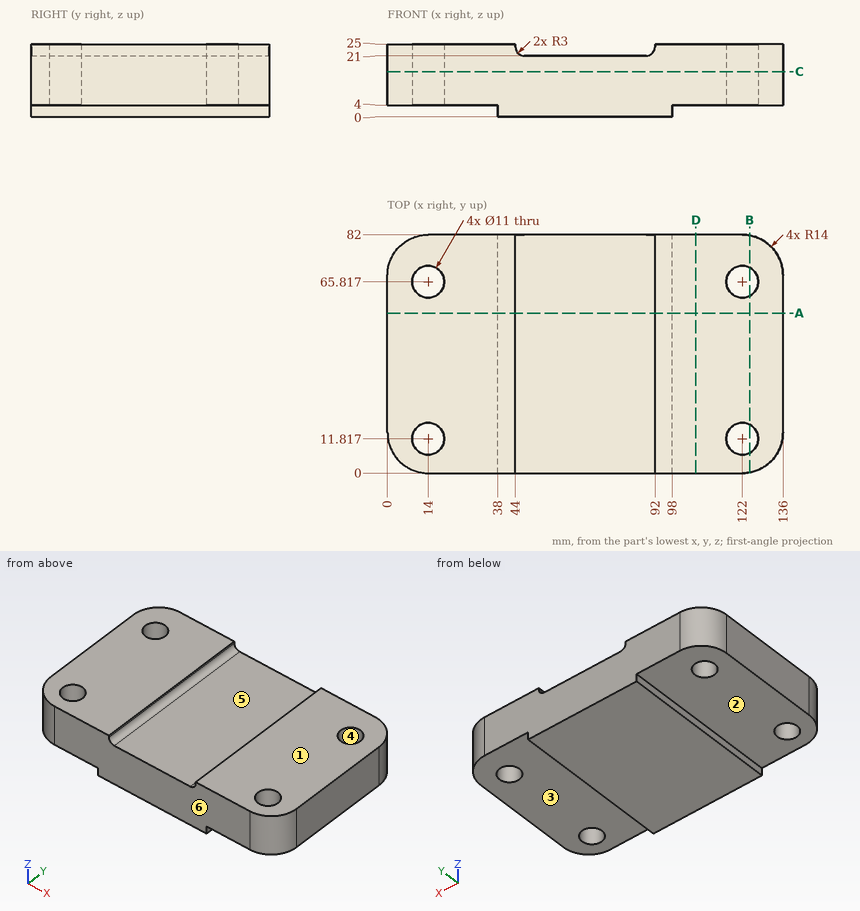
Could you check a few things on this drawing? It's one solid part, dimensions in mm from its lowest x, y, z. A direction names the side the tool comes from. Coordinates: 2 decimals unless noted, no trailing zeros. Order: outer loops, then holes, each group sorted by start corner. A loop starts at its lowest first (then second) coordinate and runs counter-clockwise, first axis right, second up. Notation, with made-up numbers: M -34,88 L -24,88 A33 ccw -24,121 Z; hole C 63.25,-14.75 d3. An arc over 180 degrees is marked long. Use a Markdown table: item, result. Add a question column.
Q1. I'm going to push flat-ended pins straight in: pin 1 (2 mm diameter, centred on y = 22, z = 2, fed in from -X); pin 2 (2 mm diameter, centred on x = 17.5, y = 53, fed in from -Z); pin 3 (1.2 mm diameter, centred on y = 36, z = 1.5, fed in from +X). Where does each tip first touch, or does it pass through?
Q2. I want a section at B-B on x = 124.5. List the corners of the cut face in (y, z) for me (1 decimal).
Q3. I want a section at C-C on z = 15.5. List the corners of the cut face in (x, y) for me.
Q4. We'd pull the mould along Y, two halves only. Please class the marked faces 4, 5 and 6: pulls with the +Y half, pulls with the -Y half, needs draft (parallel to the pull), parting line crosses it, or undercut.
Q5. I want a section at D-D on x = 106. List the corners of the cut face in (y, z) for me.
Q6. I want a section at A-A on y = 55. List the corners of the cut face in (x, z) for me, then the cut area to 3 significant figures.
Q7. Which directions (+Z, -Z, +X, -X, +Y, -Y) give clear straight access to the entire face, cutting with the end or side of a thin tool? Please do the marked faces 1, 2 and 3.
Q8. If I drill on L1, parallel to Y at x = 14, z = 14.25; L2, parallel to X at y = 10, z = 9.5; L3, parallel to Y at x = 16, z = 19 (1 decimal), over which ranges is the centre line in solid material (lowest first)?
Checked values:
| question | item | result |
|---|---|---|
| 1 | pin 1 | x = 38 |
| 1 | pin 2 | z = 4 |
| 1 | pin 3 | x = 98 |
| 2 | outline | M 0.2,4 L 6.9,4 L 6.9,25 L 0.2,25 Z; M 16.7,4 L 60.9,4 L 60.9,25 L 16.7,25 Z; M 70.7,4 L 81.8,4 L 81.8,25 L 70.7,25 Z |
| 3 | outline | M 0,14 A14 ccw 14,0 L 122,0 A14 ccw 136,14 L 136,68 A14 ccw 122,82 L 14,82 A14 ccw 0,68 Z; hole C 14,11.82 d11; hole C 14,65.82 d11; hole C 122,11.82 d11; hole C 122,65.82 d11 |
| 4 | face 4 | undercut |
| 4 | face 5 | needs draft |
| 4 | face 6 | pulls with the -Y half |
| 5 | outline | M 0,4 L 82,4 L 82,25 L 0,25 Z |
| 6 | outline | M 0,4 L 38,4 L 38,0 L 98,0 L 98,4 L 136,4 L 136,25 L 92,25 L 92,24 A3 cw 89,21 L 47,21 A3 cw 44,24 L 44,25 L 0,25 Z |
| 6 | area | 2,910 mm² |
| 7 | face 1 | +Z, +X, -X, +Y, -Y |
| 7 | face 2 | -Z, -X, +Y, -Y |
| 7 | face 3 | -Z, +X, +Y, -Y |
| 8 | L1 | 0 to 6.32, 17.32 to 60.32, 71.32 to 82 |
| 8 | L2 | 0.58 to 8.81, 19.19 to 116.81, 127.19 to 135.42 |
| 8 | L3 | 0 to 6.7, 16.9 to 60.7, 70.9 to 82 |
